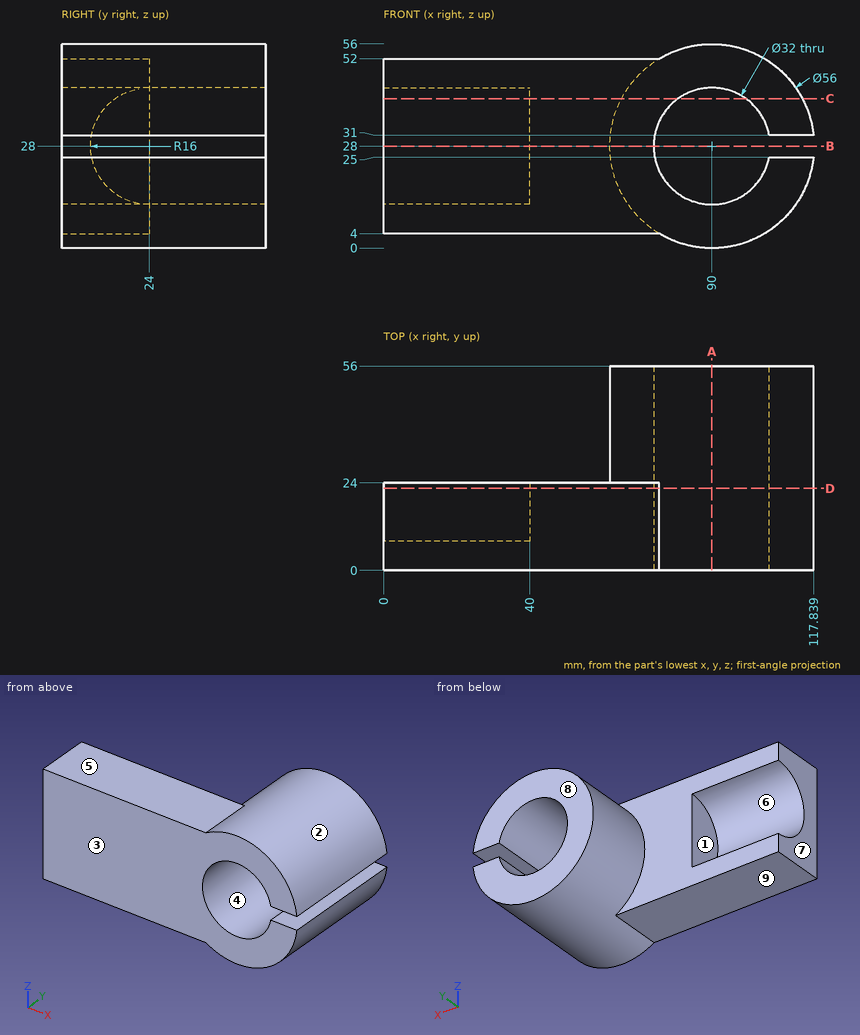
The drawing under review shows one solid part. Ordinate dimensions are in mm from its lowest x, y, z. A direction names the side the tool comes from. Coordinates: 2 decimals unless noted, no trailing zeros. Order: outer loops, then holes, each group sorted by start corner. A loop starts at its lowest first (then second) coordinate and runs counter-clockwise, first axis right, second up. Notation, with made-up numbers: (-11, 69) -> (-5, 69) arc R18 cw to (-5, 95) -> close; hole circle Ø9 at (82, 36.25). An arc over 180 degrees is marked (long way). Use CSV: the item, a comma, the result in double quotes. Start each with the question number.
Item 1: We need section C-C, the plane z = 41. Give the boundary of the cut face in (x, y).
Item 2: Draft analysis for pull direction X (two halves, no side actions). For the marked faces 1, 2, 3 and 4, state which applies: pulls with the +X half, pulls with the -X half, needs draft (parallel to the pull), parting line crosses it, or undercut.
Item 3: For the marked faces 5, 6, 7, 8 and 9, list the 3-axis set-ups (+Z, -Z, +X, -X, +Y, -Y) from which the entire face can be reached by the end or side of a thin tool; tool diameter is ignored.
Item 4: Wall thickness on probe 1 along Z at (x, y) = (90, 17); probe 2 along Z at (x, y) = (63, 5.5); probe 3 along Y at (x, z) = (16, 8.5): over which ranges is each line inside the solid? List them lowest first.
Item 5: Insertion check: pin 1 (12 mm diameter, centred on x = 52, y = 14.5, fed in from -Z); pin 2 (6 mm diameter, centred on x = 112.5, y = 26, fed in from +Z); pin 3 (6 mm diameter, centred on y = 20, z = 24, fed in from -X). Each pin has a flat end and moves straight along its axis. Give the tip position at first contact, or say it passes through.
Item 6: We need section D-D, the plane y = 22.5. Give the boundary of the cut face in (x, z).
Item 7: We need section A-A, the plane x = 90. Give the boundary of the cut face in (y, z), then the cut area to 3 significant figures.
Item 8: We need section B-B, the plane z = 28. Give the boundary of the cut face in (x, y).
Derived:
1,outline,"(0, 0) -> (80.67, 0) -> (80.67, 56) -> (65.2, 56) -> (65.2, 24) -> (40, 24) -> (40, 14.67) -> (0, 14.67) -> close; (99.33, 0) -> (114.8, 0) -> (114.8, 56) -> (99.33, 56) -> close"
2,face 1,"pulls with the -X half"
2,face 2,"parting line crosses it"
2,face 3,"needs draft"
2,face 4,"undercut"
3,face 5,"+Z, -X, +Y, -Y"
3,face 6,"-X, +Y"
3,face 7,"+Z, -Z, -X, +Y, -Y"
3,face 8,"+Z, -Z, +X, -X, +Y"
3,face 9,"-Z, -X, +Y, -Y"
4,probe 1,"z = 0 to 12, 44 to 56"
4,probe 2,"z = 4 to 52"
4,probe 3,"y = 0 to 24"
5,pin 1,"stops at z = 4"
5,pin 2,"stops at z = 48.09"
5,pin 3,"stops at x = 40"
6,outline,"(0, 4) -> (75.58, 4) arc R28 ccw to (117.84, 25) -> (105.72, 25) arc R16 cw (long way) to (105.72, 31) -> (117.84, 31) arc R28 ccw to (75.58, 52) -> (0, 52) -> (0, 43.93) -> (40, 43.93) -> (40, 12.07) -> (0, 12.07) -> close"
7,outline,"(0, 0) -> (56, 0) -> (56, 12) -> (0, 12) -> close; (0, 44) -> (56, 44) -> (56, 56) -> (0, 56) -> close"
7,area,"1,340 mm^2"
8,outline,"(0, 0) -> (74, 0) -> (74, 56) -> (62, 56) -> (62, 24) -> (40, 24) -> (40, 8) -> (0, 8) -> close"
